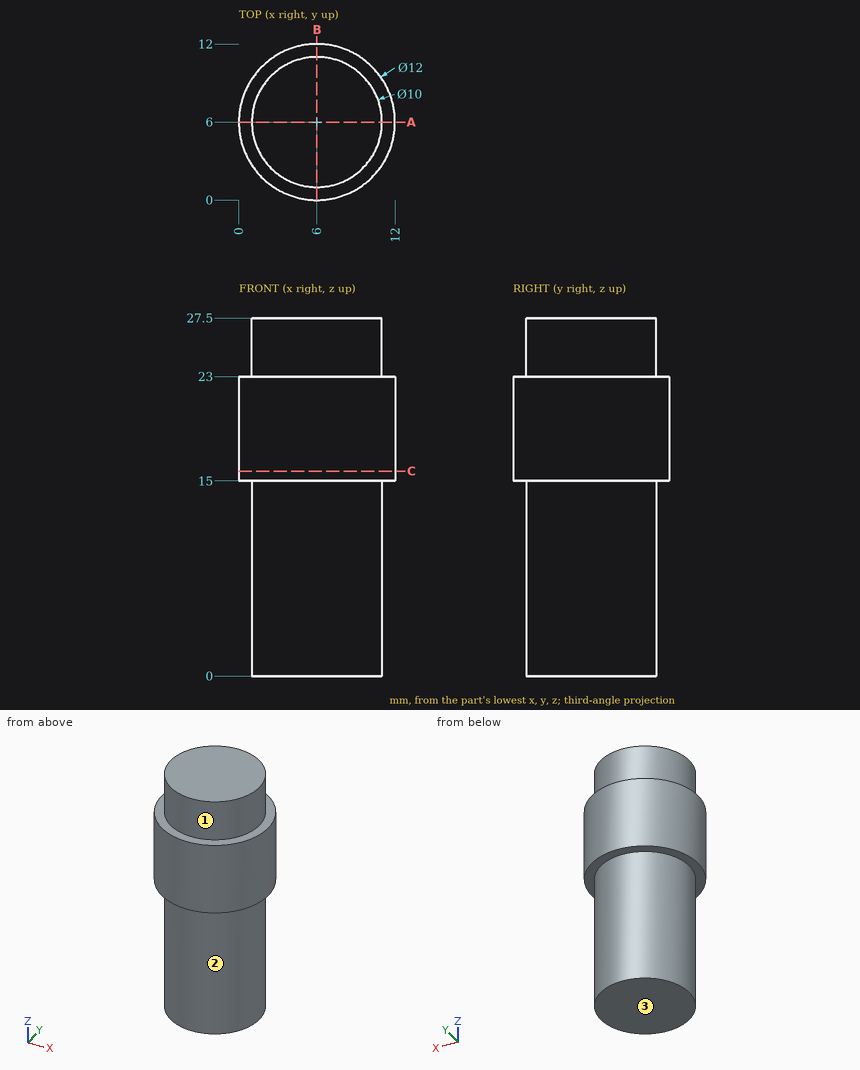
Source: three-view drawing plus pictorial views. Frame: mm from the lowest corner of the part. A direction names the side the tool comes from. Give positions to 0.01 mm unless a question says otherwise; leave off trailing zeros. Write each loop counter-clockwise with the first axis right and the second up, starting at its lowest first coordinate (ties: lowest second). Pieces come first, ordered by that corner, then holes. Notation, with made-up numbers: (-8.75, -15) - (-0.75, -15) arc R32 cw to (-0.75, 17) - close; hole circle Ø2 at (88.25, 82.5). An arc over 180 degrees is marked (long way). Write item = value, one per line. Start each with the question number.
Q1. Reachability of the marked faces 1, 2 and 3 from +Z, -Z, +X, -X, +Y, -Y: full face, straight path, thin tool, end or side. Return the list, or none.
Q2. Material intervals for probe 1 along Z at (x, y) = (5.75, 11.5); probe 2 along X at (y, z) = (6.25, 19); probe 3 along Y at (x, z) = (9, 3.5), sorted ascending.
Q3. Pin query (flat end, axial travel): pin 1 Ø2 at (y, z) = (4.5, 22) entering from +X; pin 2 Ø6 at (y, z) = (1.5, 12) entering from +X; pin 3 Ø1 at (y, z) = (9.5, 21) entering from +X. Return the tip coordinate at first contact, or that it passes through.
Q4. Cut plane A-A, the plane y = 6. Return loops of the section in (x, z).
Q5. Cut plane C-C, the plane z = 15.75. Return loops of the section in (x, y).
Computed values:
q1.face_1 = +Z
q1.face_2 = -Z
q1.face_3 = -Z, +X, -X, +Y, -Y
q2.probe_1 = 15 to 23
q2.probe_2 = 0.01 to 11.99
q2.probe_3 = 2 to 10
q3.pin_1 = 11.98
q3.pin_2 = 10.77
q3.pin_3 = 11.2
q4.outline = (0, 15) - (1, 15) - (1, 0) - (11, 0) - (11, 15) - (12, 15) - (12, 23) - (11, 23) - (11, 27.5) - (1, 27.5) - (1, 23) - (0, 23) - close
q5.outline = circle Ø12 at (6, 6)
